The figure shows three views and two pictorial views of one solid part (mm, origin at its lowest corner). Answer the questions. A direction names the side the tool comes from. Round coordinates to 2 decimals unless told otherwise and drop trailing zeros. Write each loop counter-clockwise with the first axis right and the second up, starting at its lowest first coordinate (ties: lowest second). Pieces come first, ordered by that corner, then holes.
Item 1: A tool of negligible diameter and unlimited length cuts with its end or side. For the marked faces 1, 2 and 3, from which of +Z, -Z, +X, -X, +Y, -Y can it reach the whole face along a straight path? Write none if from no direction.
Item 2: Find the intervals of material crossed by probe 1 along Y at (x, z) = (25, 21.5); probe 2 along Y at (x, z) = (332, 25); probe 3 along Y at (x, z) = (24, 23.5), in increasing order.
Item 3: Find section B-B on x = 396.5. Give the vertices of the cut face in (y, z), then the cut area to 3 significant figures.
Item 4: Each of these flat-tipped pins is pushed along its axis until it touches: pin 1 (5 mm diameter, centred on x = 201.5, z = 24, fed in from -Y); pin 2 (20 mm diameter, centred on y = 15, z = 20, fed in from +X); pin 3 (4 mm diameter, centred on x = 312, z = 6, fed in from +Y). Where does it stop, or does it pass through?
Item 5: Find section D-D on y = 89. Give the vertices of the cut face in (x, z), then the cut area to 3 significant figures.
Item 6: Find section C-C on z = 27. Give the number of separate pieces and of enclosed holes in the cut face, then the cut area to 3 significant figures.
Item 7: Find section A-A on y = 320. Give the vertices of the cut face in (x, z).
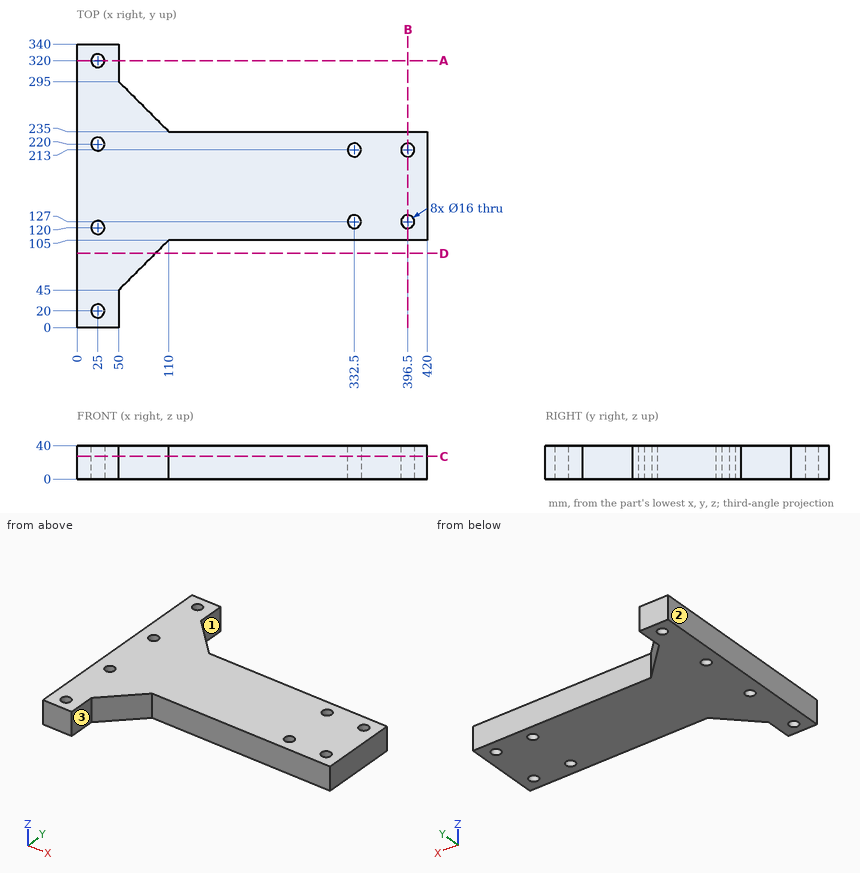
Check values:
1. face 1: +Z, -Z, +X, +Y
1. face 2: +Z, -Z, -X, +Y, -Y
1. face 3: +Z, -Z, +X, -Y
2. probe 1: y = 0 to 12, 28 to 112, 128 to 212, 228 to 312, 328 to 340
2. probe 2: y = 105 to 119.02, 134.98 to 205.02, 220.98 to 235
2. probe 3: y = 0 to 12.06, 27.94 to 112.06, 127.94 to 212.06, 227.94 to 312.06, 327.94 to 340
3. outline: (105, 0) - (119, 0) - (119, 40) - (105, 40) - close; (135, 0) - (205, 0) - (205, 40) - (135, 40) - close; (221, 0) - (235, 0) - (235, 40) - (221, 40) - close
3. area: 3,920 mm2
4. pin 1: stops at y = 105
4. pin 2: stops at x = 50
4. pin 3: stops at y = 235
5. outline: (0, 0) - (94, 0) - (94, 40) - (0, 40) - close
5. area: 3,760 mm2
6. separate pieces: 1
6. enclosed holes: 8
6. area: 67,100 mm2
7. outline: (0, 0) - (17, 0) - (17, 40) - (0, 40) - close; (33, 0) - (50, 0) - (50, 40) - (33, 40) - close
